Part print with two shaded views. Sizes in mm from the minimum x, y, z corner. A direction names the side the tool comes from. Coordinates: 2 decimals unless noted, no trailing zeros. Write each loop counter-clockwise with the first axis right and the second up, starting at its lowest first coordinate (ties: lowest second). Pieces come first, ordered by that corner, then holes. Notation, with made-up numbers: M 72,-31 L 91,-31 A26 cw 91,-16 Z; hole C 3.5,6.5 d1. An arc over 180 degrees is marked long. One line per question, with ' | ' between items. Start each with the question number.
(1) Flat gauge pins, fed straight in: pin 1 Ø10 at (y, z) = (4.5, 17) entering from -X; pin 2 Ø12 at (y, z) = (12, 35) entering from -X; pin 3 Ø6 at (x, z) = (18.5, 25) entering from +Y. Where does each tip first touch, or does it go through?
(2) Cut at D-D (z = 5.5). Write the cut outline in (x, y).
(3) Wall check: probe 1 along Z at (x, y) = (18, 26.5); probe 2 along X at (y, z) = (36, 21); probe 3 along Y at (x, z) = (33, 35). Give the ranges that are in metal, low to high.
(4) Cut at B-B (z = 35). Write the cut outline in (x, y).
(5) Cut at C-C (y = 15.5). Write the cut outline in (x, z), plus the area to 3 significant figures.
(6) Cut at A-A (x = 29.5). Write the cut outline in (y, z).
(7) Tool access for the marked faces 1 and 2: list every direction of +Z, -Z, +X, -X, +Y, -Y with a clear straight run to the whole face (end or side of a thin tool).
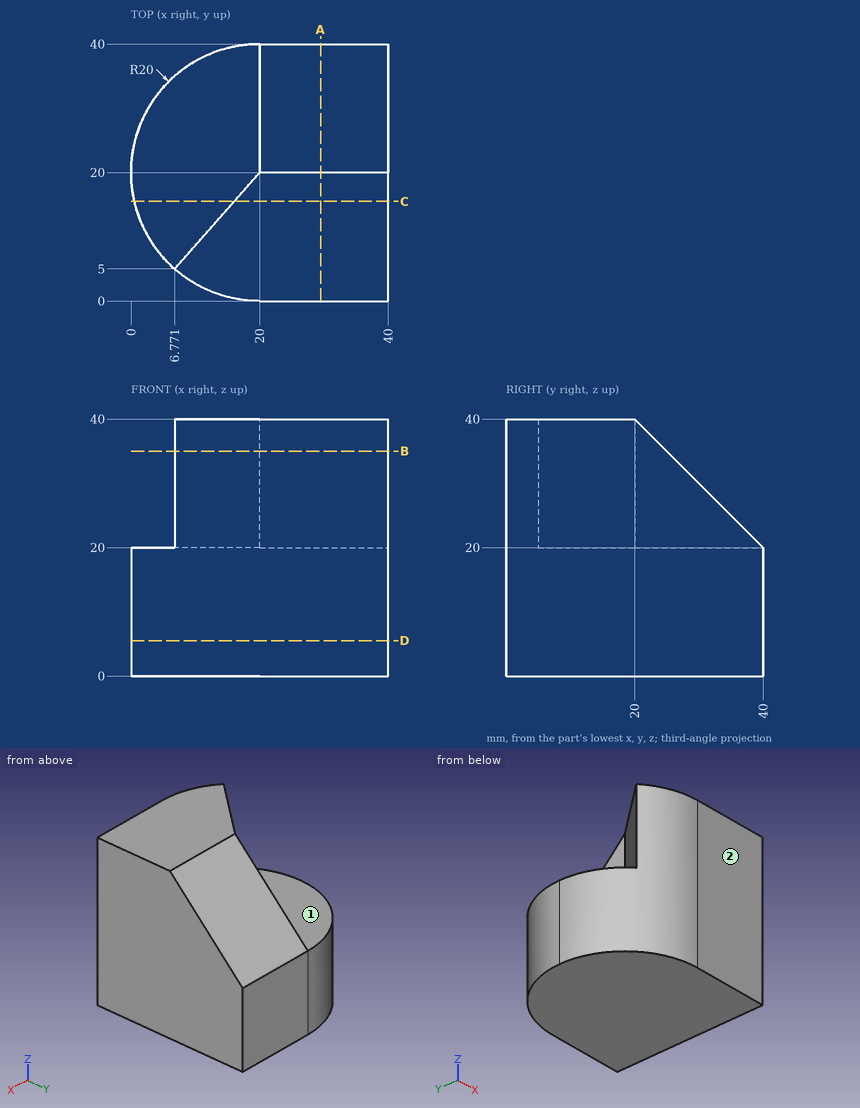
Filled in:
1) pin 1: x = 2.98 | pin 2: x = 7.65 | pin 3: y = 37.6
2) outline: M 20,0 L 40,0 L 40,40 L 20,40 A20 ccw Z
3) probe 1: 0 to 20 | probe 2: 20 to 40 | probe 3: 0 to 25
4) outline: M 6.77,5 A20 ccw 20,0 L 40,0 L 40,25 L 20,25 L 20,20 Z
5) outline: M 0.51,0 L 40,0 L 40,40 L 16.03,40 L 16.03,20 L 0.51,20 Z | area: 1,270 mm²
6) outline: M 0,0 L 40,0 L 40,20 L 20,40 L 0,40 Z
7) face 1: +Z, -X, +Y | face 2: +Z, -Z, +X, -X, -Y
